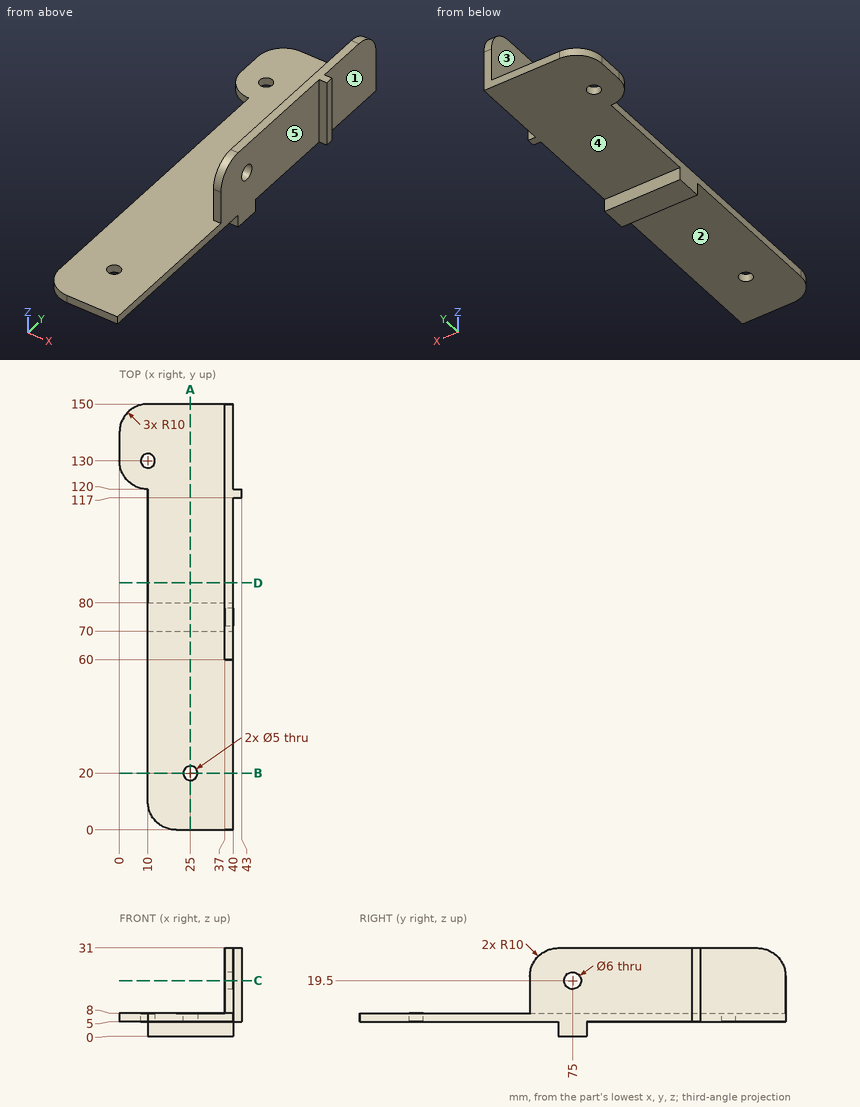
Geometry: see drawing. Coordinates: mm, zero at the bounding-box minimum. A direction names the side the tool comes from. Give positions to 0.01 mm unless a question says otherwise; leave off trailing zeros. Write each loop counter-clockwise with the first axis right and the second up, starting at its lowest first coordinate (ties: lowest second). Pieces come first, ordered by that corner, then holes. Notation, with made-up numbers: M 29.5,76.25 L 87.5,76.25 A15 cw 87.5,84.25 Z; hole C -21,66 d9. An arc over 180 degrees is marked long. Answer as a JSON object with one key per item and string values.
Q1. Ray query, line 1 along Y through (x, z) = (25, 6.35); line 2 along Z through (x, y) = (21.5, 66.5); line 3 along X through (y, z) = (130, 6.5). Return the intervals inside material, ascending.
Geometry check:
{"line 1": "y = 0 to 17.5, 22.5 to 150", "line 2": "z = 5 to 8", "line 3": "x = 0 to 7.5, 12.5 to 40"}
Q2. Cut plane B-B, the plane y = 20. Return the cut outline in (x, z), then the cut area to 3 significant figures.
Geometry check:
{"outline": "M 10,5 L 22.5,5 L 22.5,8 L 10,8 Z; M 27.5,5 L 40,5 L 40,8 L 27.5,8 Z", "area": "75.0 mm^2"}
Q3. Access query for the marked faces 1, 2, 3, 4 and 5. Directions: +Z, -Z, +X, -X, +Y, -Y. A direction counts if a zero-diameter tool reaches every point of the face in a straight line with its end or side. Return the directions, or none.
Geometry check:
{"face 1": "+Z, -Z, +X, +Y", "face 2": "-Z, +X, -X, -Y", "face 3": "+Z, -X, +Y, -Y", "face 4": "-Z, +X, -X, +Y", "face 5": "+Z, -Z, +X, -Y"}
Q4. Contact query for flat-ended pins moving along their axis: P1, Ø21.5, axis at x = 12, y = 104, coming from the -Z side; P2, Ø2.5, axis at x = 28.5, z = 3, coming from the -Y side; P3, Ø1.5, axis at x = 30, z = 1.5, coming from the +Y side; P4, Ø4.5, axis at x = 25, y = 20, coming from the -Z side. Output: stop coordinate, or through.
Geometry check:
{"P1": "stops at z = 5", "P2": "stops at y = 70", "P3": "stops at y = 80", "P4": "passes through"}
Q5. Cut plane A-A, the plane x = 25. Return the cut outline in (y, z), then the cut area to 3 significant figures.
Geometry check:
{"outline": "M 0,5 L 17.5,5 L 17.5,8 L 0,8 Z; M 22.5,5 L 70,5 L 70,0 L 80,0 L 80,5 L 150,5 L 150,8 L 22.5,8 Z", "area": "485 mm^2"}
Q6. Cut plane C-C, the plane z = 19.5. Return the cut outline in (x, y).
Geometry check:
{"outline": "M 37,60 L 40,60 L 40,72 L 37,72 Z; M 37,78 L 40,78 L 40,117 L 43,117 L 43,120 L 40,120 L 40,150 L 37,150 Z"}
Q7. Cut plane D-D, the plane y = 87. Return the cut outline in (x, z).
Geometry check:
{"outline": "M 10,5 L 40,5 L 40,31 L 37,31 L 37,8 L 10,8 Z"}
